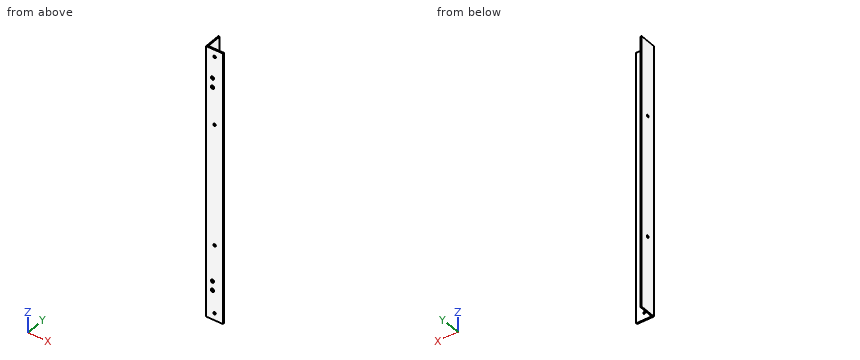
from build123d import *

# Parameters (mm, degrees)
EXTRUSION1_DEPTH = 325
ESQUISSE2_R      = 1.5
ESQUISSE2_R_2    = 2
EXTRUSION2_DEPTH = 300
ESQUISSE3_R      = 1.5
EXTRUSION3_DEPTH = 10


with BuildPart() as part:
    # Esquisse1 → Extrusion1 (new body)
    with BuildSketch(Plane.XY):
        Polygon((-17.43168638, 4.773368421), (-17.43168638, -15.226631579), (2.56831362, -15.226631579), (2.56831362, -13.726631579), (-15.93168638, -13.726631579), (-15.93168638, 4.773368421), align=None)
    extrude(amount=EXTRUSION1_DEPTH)

    # Esquisse2 → Extrusion2 (cut)
    with BuildSketch(Plane(origin=(0, -13.726631579, 0), x_dir=(-1, 0, 0), z_dir=(0, 1, 0))):
        with Locations((7.43168638, 8.5)):
            Circle(ESQUISSE2_R)
        with Locations((7.43168638, 316.5)):
            Circle(ESQUISSE2_R)
        with Locations((9.93168638, 35)):
            Circle(ESQUISSE2_R_2)
        with Locations((9.93168638, 46)):
            Circle(ESQUISSE2_R_2)
        with Locations((9.93168638, 290)):
            Circle(ESQUISSE2_R_2)
        with Locations((9.93168638, 279)):
            Circle(ESQUISSE2_R_2)
        with Locations((7.43168638, 235)):
            Circle(ESQUISSE2_R)
        with Locations((7.43168638, 90)):
            Circle(ESQUISSE2_R)
    extrude(amount=-EXTRUSION2_DEPTH, mode=Mode.SUBTRACT)

    # Esquisse3 → Extrusion3 (cut)
    with BuildSketch(Plane.ZY.offset(17.43168638)):
        with Locations(Location((235, -5.226631579, 0), (0, 0, 270))):
            Circle(ESQUISSE3_R)
        with Locations(Location((90, -5.226631579, 0), (0, 0, 270))):
            Circle(ESQUISSE3_R)
    extrude(amount=-EXTRUSION3_DEPTH, mode=Mode.SUBTRACT)


solid = part.part
Read the model definition and answer for the solid it produces. Units are mm, in the model's axes. Coordinates: 2 decimals unless noted, no trailing zeros. Loops run counter-clockwise (first coordinate to the right, second up) from the corner with the lowest first, then second, coordinate; pieces in that order, holes last. Notation, with made-up numbers: (-27, -24.75) - (32, -24.75) arc R36 cw to (32, 9.25) - close; hole circle Ø2 at (15, 65). An arc over 180 degrees is marked (long way). Answer in a Markdown table with one row per item.
Q1. Find section B-B on y = 2. Write down the section's boundary in (x, z).
Here are the results:
| item | result |
|---|---|
| outline | (-17.43, 0) - (-15.93, 0) - (-15.93, 325) - (-17.43, 325) - close |
Q2. Find section C-C on x = -0.5. Write down the section's boundary in (y, z).
Here are the results:
| item | result |
|---|---|
| outline | (-15.23, 0) - (-13.73, 0) - (-13.73, 325) - (-15.23, 325) - close |
Q3. Find section A-A on z = 175. Write down the section's boundary in (x, y).
Here are the results:
| item | result |
|---|---|
| outline | (-17.43, -15.23) - (2.57, -15.23) - (2.57, -13.73) - (-15.93, -13.73) - (-15.93, 4.77) - (-17.43, 4.77) - close |
Q4. Given P1, Ø2.5, axis at y = -5.23, z = 235, coming from the +X side; P2, Ø1.5, axis at x = -1, z = 56, coming from the +Y side; P3, Ø1.5, axis at y = -12, z = 81, coming from the +X side, each flat-ended and moving along its own axis, determine where each tip first touches the part or whether it passes through.
Here are the results:
| item | result |
|---|---|
| P1 | passes through |
| P2 | stops at y = -13.73 |
| P3 | stops at x = -15.93 |
Q5. Straight lines are drawn through the part: line 1 along X through (y, z) = (-14.4, 279); line 2 along Y through (x, z) = (-7, 24); line 3 along X through (y, z) = (-8.75, 137). For each, find the intervals that lie inside material, in ascending order. Write a range as [from, to].
Here are the results:
| item | result |
|---|---|
| line 1 | x = [-17.43, -11.93], [-7.93, 2.57] |
| line 2 | y = [-15.23, -13.73] |
| line 3 | x = [-17.43, -15.93] |
